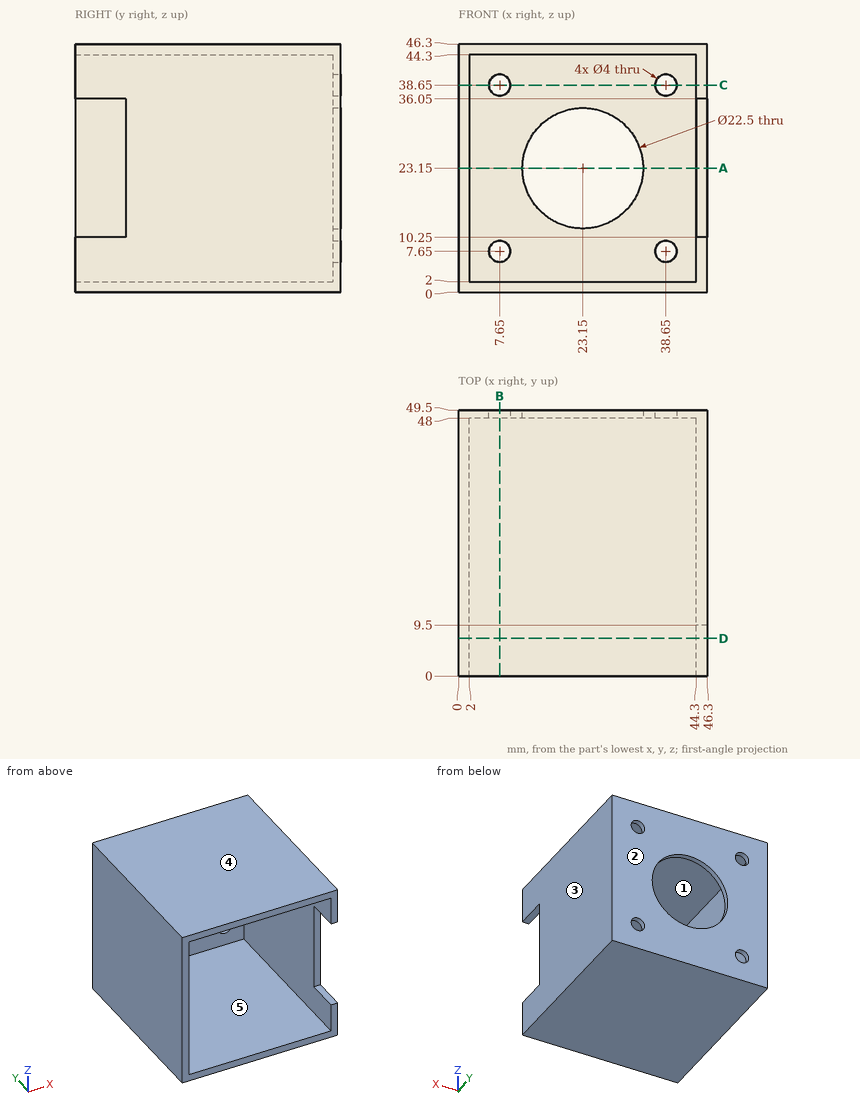
Drawing for the job (mm, zero at the part's lowest x, y, z). A direction names the side the tool comes from. Round coordinates to 2 decimals unless told otherwise and drop trailing zeros. Loops run counter-clockwise (first coordinate to the right, second up) from the corner with the lowest first, then second, coordinate; pieces in that order, holes last. Notation, with made-up numbers: (70.5, -19) - (110.5, -19) arc R16 ccw to (110.5, -3) - close; hole circle Ø9 at (63.5, 63.5). An arc over 180 degrees is marked (long way). Return JSON: item names as keys, results as strings. Group by question number.
Q1. Band-saw the part on B-B on x = 7.65. Give the cut face in (y, z), plus the area to 3 significant figures.
Q2. Band-saw the part on C-C on z = 38.65. Give the cut face in (x, y).
Q3. Tool access for the marked faces 4 and 5: list every direction of +Z, -Z, +X, -X, +Y, -Y with a clear straight run to the whole face (end or side of a thin tool).
Q4. Band-saw the part on A-A on z = 23.15. Give the cut face in (x, y).
Q5. Two-plate mould, pull along X, no slides. Class the marked faces 1, 2 and 3: +X half, -X half, draft (parallel to the pull), parting line (faces both ways), or undercut.
Q6. Drill centre lines: line 1 along X through (y, z) = (49, 7.65); line 2 along X through (y, z) = (15, 31). Where is each one in solid material? Low to high. Write a range as [from, to].
Q7. Band-saw the part on D-D on y = 7. Give the cut face in (x, z).
Q8. Flat gauge pins, fed straight in: pin 1 Ø6.5 at (x, z) = (7.65, 7.65) entering from -Y; pin 2 Ø18 at (x, z) = (23.15, 23.15) entering from +Y; pin 3 Ø1 at (x, z) = (45, 25.5) entering from -Y. Where does each tip first touch, or does it go through?
Solutions:
{
 "1": {"outline": "(0, 0) - (49.5, 0) - (49.5, 5.65) - (48, 5.65) - (48, 2) - (0, 2) - close; (0, 44.3) - (48, 44.3) - (48, 40.65) - (49.5, 40.65) - (49.5, 46.3) - (0, 46.3) - close; (48, 9.65) - (49.5, 9.65) - (49.5, 36.65) - (48, 36.65) - close", "area": "249 mm^2"},
 "2": {"outline": "(0, 0) - (2, 0) - (2, 48) - (5.65, 48) - (5.65, 49.5) - (0, 49.5) - close; (9.65, 48) - (36.65, 48) - (36.65, 49.5) - (9.65, 49.5) - close; (40.65, 48) - (44.3, 48) - (44.3, 0) - (46.3, 0) - (46.3, 49.5) - (40.65, 49.5) - close"},
 "3": {"face 4": "+Z, +X, -X, +Y, -Y", "face 5": "-Y"},
 "4": {"outline": "(0, 0) - (2, 0) - (2, 48) - (11.9, 48) - (11.9, 49.5) - (0, 49.5) - close; (34.4, 48) - (44.3, 48) - (44.3, 9.5) - (46.3, 9.5) - (46.3, 49.5) - (34.4, 49.5) - close"},
 "5": {"face 1": "undercut", "face 2": "draft", "face 3": "+X half"},
 "6": {"line 1": "x = [0, 5.65], [9.65, 36.65], [40.65, 46.3]", "line 2": "x = [0, 2], [44.3, 46.3]"},
 "7": {"outline": "(0, 0) - (46.3, 0) - (46.3, 10.25) - (44.3, 10.25) - (44.3, 2) - (2, 2) - (2, 44.3) - (44.3, 44.3) - (44.3, 36.05) - (46.3, 36.05) - (46.3, 46.3) - (0, 46.3) - close"},
 "8": {"pin 1": "stops at y = 48", "pin 2": "passes through", "pin 3": "stops at y = 9.5"}
}
